Work out the finished part from the listing and answer in its coordinate system (mm). A direction names the side the tool comes from. Round coordinates to 2 decimals unless told otherwise and drop trailing zeros. Loops run counter-clockwise (first coordinate to the right, second up) from the corner with the lowest first, then second, coordinate; pieces in that order, holes last.
```python
from build123d import *

# Parameters (mm, degrees)
SKETCH057_W             = 9
SKETCH057_H             = 19
SKETCH057_R             = 1.3375
PAD030_DEPTH            = 9
SKETCH058_W             = 9
SKETCH058_H             = 9
PAD031_DEPTH            = 15.5
SKETCH059_R             = 2.5
POCKET026_DEPTH         = 19.001
BODY013_PLACEMENT_ANGLE = 90


with BuildPart() as part:
    # Sketch057 → Pad030 (new body)
    with BuildSketch(Plane.XY):
        with Locations((4.5, 9.5)):
            Rectangle(SKETCH057_W, SKETCH057_H)
        with Locations((4.5, 5)):
            Circle(SKETCH057_R, mode=Mode.SUBTRACT)
    extrude(amount=PAD030_DEPTH)

    # Sketch058 (on Face7 of Pad030) → Pad031 (join)
    with BuildSketch(Plane.XY.offset(9)):
        with Locations((4.5, 14.5)):
            Rectangle(SKETCH058_W, SKETCH058_H)
    extrude(amount=PAD031_DEPTH)

    # Sketch059 (on Face11 of Pad031) → Pocket026 (cut, through all)
    with BuildSketch(Plane(origin=(0, 19, 0), x_dir=(-1, 0, 0), z_dir=(0, 1, 0))):
        with Locations((-4.5, 20)):
            Circle(SKETCH059_R)
    extrude(amount=-POCKET026_DEPTH, mode=Mode.SUBTRACT)


with BuildPart() as part_1:
    # Body013 placement: moved
    add(part.part.moved(Location((-144, 115, 69.5))).rotate(Axis((-144, 115, 69.5), (0, 1, 0)), BODY013_PLACEMENT_ANGLE))


solid = part_1.part
```
1. Find section C-C (x = -124). Write down the section's boundary in (y, z), then the cut area to 3 significant figures.
Answer key:
outline: (125, 60.5) - (134, 60.5) - (134, 62.5) - (125, 62.5) - close; (125, 67.5) - (134, 67.5) - (134, 69.5) - (125, 69.5) - close
area: 36.0 mm2
2. Find section D-D (z = 67). Write down the section's boundary in (x, y), then the cut area to 4 significant figures.
Answer key:
outline: (-144, 115) - (-135, 115) - (-135, 125) - (-125.5, 125) - (-125.5, 134) - (-144, 134) - close; (-122.5, 125) - (-119.5, 125) - (-119.5, 134) - (-122.5, 134) - close
area: 283.5 mm2
3. Determine the mould class of faces 3 (the face through (-135, 126, 60.5)), 4 (the face through (-144, 125, 65)), 5 (the face through (-121.52, 129.56, 64.67)) for opening direction X: +X half, -X half, draft (parallel to the pull), parting line (faces both ways), or undercut.
Answer key:
face 3: draft
face 4: -X half
face 5: undercut
4. Consider probe 1 along Z at (x, y) = (-139, 120); probe 2 along Y at (x, z) = (-140.5, 65); probe 3 along X at (y, z) = (127, 65). Determine where each line is inside the solid, lowest interval first.
Answer key:
probe 1: z = 60.5 to 63.66, 66.34 to 69.5
probe 2: y = 115 to 118.66, 121.34 to 134
probe 3: x = -144 to -126.5, -121.5 to -119.5
5. Find section B-B (y = 120). Write down the section's boundary in (x, z), then the cut area to 3 significant figures.
Answer key:
outline: (-144, 60.5) - (-135, 60.5) - (-135, 63.66) - (-144, 63.66) - close; (-144, 66.34) - (-135, 66.34) - (-135, 69.5) - (-144, 69.5) - close
area: 56.9 mm2
6. Find section A-A (z = 65). Write down the section's boundary in (x, y), then the cut area to 3 significant figures.
Answer key:
outline: (-144, 115) - (-135, 115) - (-135, 118.66) - (-144, 118.66) - close; (-144, 121.34) - (-135, 121.34) - (-135, 125) - (-126.5, 125) - (-126.5, 134) - (-144, 134) - close; (-121.5, 125) - (-119.5, 125) - (-119.5, 134) - (-121.5, 134) - close
area: 241 mm2
7. Which of the six approach directions +Z, -Z, +X, -X, +Y, -Y give full straight-line access (tool end or side, diameter ignored) to faces 1 (the face through (-127, 125, 65)), 2 (the face through (-140, 115, 65))?
Answer key:
face 1: +Z, -Z, +X, -Y
face 2: +Z, -Z, +X, -X, -Y
